Design review of the part shown in the three views and the two pictorial views. Dimensions are in mm from the part's minimum x, y and z. Coordinates: 2 decimals unless noted, no trailing zeros. Loops run counter-clockwise (first coordinate to the right, second up) from the corner with the lowest first, then second, coordinate; pieces in that order, holes last.
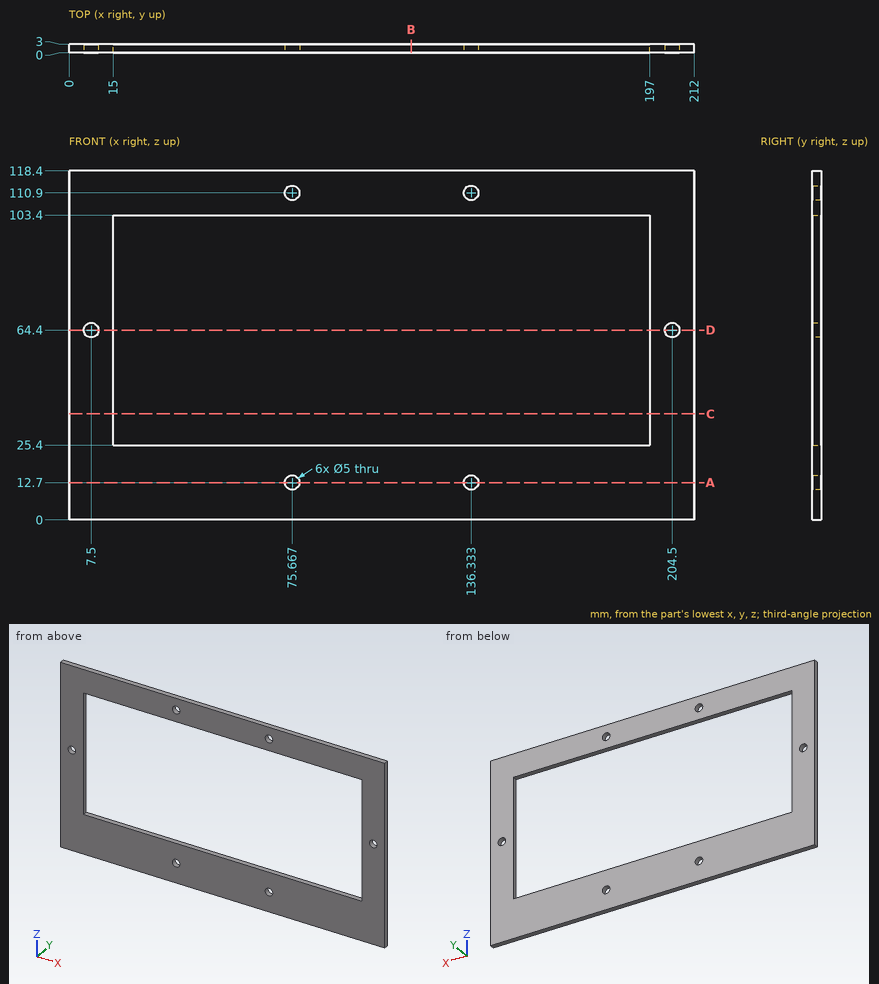
Q1. Consider section D-D (z = 64.4). State the section outline as (x, y) points.
Q2. Consider section A-A (z = 12.7). State the section outline as (x, y) points, then the cut area to 3 significant figures.
Q3. Consider section B-B (x = 116). State the section outline as (y, z) points, then the cut area to 3 significant figures.
Q4. Consider section C-C (z = 36). State the section outline as (x, y) points, then the cut area to 3 significant figures.
Q5. For pin 1 Ø4 at (x, z) = (131, 28.5) entering from -Y, flat-tipped, find the tip position at first contact; note if it passes through.
Q6. Wall thickness on probe 1 along X at (y, z) = (0.4, 64); probe 2 along X at (y, z) = (1.55, 110.9); probe 3 along Z at (x, y) = (55, 2.1): over which ranges is each line inside the solid? List them lowest first.
Model answer:
1. outline: (0, 0) - (5, 0) - (5, 3) - (0, 3) - close; (10, 0) - (15, 0) - (15, 3) - (10, 3) - close; (197, 0) - (202, 0) - (202, 3) - (197, 3) - close; (207, 0) - (212, 0) - (212, 3) - (207, 3) - close
2. outline: (0, 0) - (73.17, 0) - (73.17, 3) - (0, 3) - close; (78.17, 0) - (133.83, 0) - (133.83, 3) - (78.17, 3) - close; (138.83, 0) - (212, 0) - (212, 3) - (138.83, 3) - close
2. area: 606 mm2
3. outline: (0, 0) - (3, 0) - (3, 25.4) - (0, 25.4) - close; (0, 103.4) - (3, 103.4) - (3, 118.4) - (0, 118.4) - close
3. area: 121 mm2
4. outline: (0, 0) - (15, 0) - (15, 3) - (0, 3) - close; (197, 0) - (212, 0) - (212, 3) - (197, 3) - close
4. area: 90.0 mm2
5. pin 1: passes through
6. probe 1: x = 0 to 5.03, 9.97 to 15, 197 to 202.03, 206.97 to 212
6. probe 2: x = 0 to 73.17, 78.17 to 133.83, 138.83 to 212
6. probe 3: z = 0 to 25.4, 103.4 to 118.4
